```python
from build123d import *

# Parameters (mm, degrees)
SKETCH1_W                                       = 25
SKETCH1_H                                       = 51.4
BOSS_EXTRUDE1_DEPTH                             = 28.4
SKETCH2_W                                       = 47.3
SKETCH2_H                                       = 27.1
CUT_EXTRUDE1_DEPTH                              = 147
BOSS_EXTRUDE2_DEPTH                             = 11.9
BOSS_EXTRUDE2_DEPTH_BACK                        = 2
SKETCH4_W                                       = 25
SKETCH4_H                                       = 59.6
SKETCH5_W                                       = 55.6
SKETCH5_H                                       = 9.9
CUT_EXTRUDE5_DEPTH                              = 57.010088377
SKETCH6_W                                       = 51.6
SKETCH6_H                                       = 2
CUT_EXTRUDE6_DEPTH                              = 57.010088377
SKETCH7_W                                       = 25
SKETCH7_H                                       = 3
BOSS_EXTRUDE3_DEPTH                             = 15
SKETCH8_W                                       = 25
SKETCH8_H                                       = 3
BOSS_EXTRUDE4_DEPTH                             = 15
CSK_FOR_M3_FLAT_HEAD_MACHINE_SCREW4_D           = 3.4
CSK_FOR_M3_FLAT_HEAD_MACHINE_SCREW4_DEPTH       = 10.4
CSK_FOR_M3_FLAT_HEAD_MACHINE_SCREW4_CSINK_D     = 6.3
CSK_FOR_M3_FLAT_HEAD_MACHINE_SCREW4_CSINK_ANGLE = 90
CSK_FOR_M3_FLAT_HEAD_MACHINE_SCREW4_TIP         = 1.021463052


with BuildPart() as part:
    # Sketch1 → Boss-Extrude1 (new body)
    with BuildSketch(Plane(origin=(0, 0, 0), x_dir=(1, 0, 0), z_dir=(0, 1, 0))):
        Rectangle(SKETCH1_W, SKETCH1_H)
    extrude(amount=BOSS_EXTRUDE1_DEPTH)

    # Sketch2 → Cut-Extrude1 (cut)
    with BuildSketch(Plane(origin=(12.5, 0, 0), x_dir=(0, 0, -1), z_dir=(1, 0, 0))):
        with Locations((0, 12.55)):
            Rectangle(SKETCH2_W, SKETCH2_H)
    extrude(amount=-CUT_EXTRUDE1_DEPTH, mode=Mode.SUBTRACT)

    # Sketch4 → Boss-Extrude2 (add, two sides: drawn at the far end of the back side and taken through both)
    with BuildSketch(Plane(origin=(0, 28.4, 0), x_dir=(1, 0, 0), z_dir=(0, 1, 0)).offset(-BOSS_EXTRUDE2_DEPTH_BACK)):
        Rectangle(SKETCH4_W, SKETCH4_H)
    extrude(amount=BOSS_EXTRUDE2_DEPTH + BOSS_EXTRUDE2_DEPTH_BACK)

    # Sketch5 → Cut-Extrude5 (cut, through all)
    with BuildSketch(Plane.ZY.offset(12.5)):
        with Locations((0, 33.35)):
            Rectangle(SKETCH5_W, SKETCH5_H)
    extrude(amount=-CUT_EXTRUDE5_DEPTH, mode=Mode.SUBTRACT)

    # Sketch6 → Cut-Extrude6 (cut, through all)
    with BuildSketch(Plane.ZY.offset(12.5)):
        with Locations((0, 39.3)):
            Rectangle(SKETCH6_W, SKETCH6_H)
    extrude(amount=-CUT_EXTRUDE6_DEPTH, mode=Mode.SUBTRACT)

    # Sketch7 → Boss-Extrude3 (add)
    with BuildSketch(Plane(origin=(0, 0, -25.7), x_dir=(-1, 0, 0), z_dir=(0, 0, -1))):
        with Locations((0, 1.5)):
            Rectangle(SKETCH7_W, SKETCH7_H)
    extrude(amount=BOSS_EXTRUDE3_DEPTH)

    # Sketch8 → Boss-Extrude4 (add)
    with BuildSketch(Plane.XY.offset(25.7)):
        with Locations((0, 1.5)):
            Rectangle(SKETCH8_W, SKETCH8_H)
    extrude(amount=BOSS_EXTRUDE4_DEPTH)

    # CSK for M3 Flat Head Machine Screw4
    with Locations(Plane(origin=(0, 3, 0), x_dir=(1, 0, 0), z_dir=(0, 1, 0))):
        with Locations((0, 33.2), (0, -33.2)):
            CounterSinkHole(CSK_FOR_M3_FLAT_HEAD_MACHINE_SCREW4_D / 2, CSK_FOR_M3_FLAT_HEAD_MACHINE_SCREW4_CSINK_D / 2, depth=CSK_FOR_M3_FLAT_HEAD_MACHINE_SCREW4_DEPTH, counter_sink_angle=CSK_FOR_M3_FLAT_HEAD_MACHINE_SCREW4_CSINK_ANGLE)
            with Locations((0, 0, -(CSK_FOR_M3_FLAT_HEAD_MACHINE_SCREW4_DEPTH + CSK_FOR_M3_FLAT_HEAD_MACHINE_SCREW4_TIP / 2))):  # 118° drill point
                Cone(0, CSK_FOR_M3_FLAT_HEAD_MACHINE_SCREW4_D / 2, CSK_FOR_M3_FLAT_HEAD_MACHINE_SCREW4_TIP, mode=Mode.SUBTRACT)


solid = part.part
```
Check sheet for the modelled part. Datum: model origin and axes. Units: mm. A direction names the side the tool comes from. Give positions to 0.01 mm unless a question says otherwise; leave off trailing zeros. Order: outer loops, then holes, each group sorted by start corner. A loop starts at its lowest first (then second) coordinate and runs counter-clockwise, first axis right, second up. Notation, with made-up numbers: (-1.75, -39.75) -> (29.25, -39.75) arc R31 ccw to (29.25, -14.75) -> close; hole circle Ø6 at (71.25, 17.25). An arc over 180 degrees is marked (long way). Return JSON: item names as keys, results as strings.
1. Cross-section at A-A, the plane y = 23.5. Record the cut outline in (x, z), plus the area to 4 significant figures.
From the geometry:
{"outline": "(-12.5, -25.7) -> (12.5, -25.7) -> (12.5, -23.65) -> (-12.5, -23.65) -> close; (-12.5, 23.65) -> (12.5, 23.65) -> (12.5, 25.7) -> (-12.5, 25.7) -> close", "area": "102.5 mm^2"}
2. Go/stop test with flat-tipped pins: P1, Ø8, axis at x = -6.5, z = -20.5, coming from the +Y side; P2, Ø7, axis at x = 0, y = 33, coming from the -Z side; P3, Ø10, axis at x = 3, y = 17, coming from the +Z side. Record where each tip stops, or that it passes through.
From the geometry:
{"P1": "y = 28.4", "P2": "z = -29.8", "P3": "z = 25.7"}
3. Mould release check, pull along Z, two halves, no side actions. Record for faces 1 (the flat face through (0, 33, -27.8)), 2 (the flat face through (0, 2, 40.7)), 3 (the flat face through (0, 40.3, 28)): +Z half, -Z half, draft (parallel to the pull), parting line (faces both ways), or undercut.
From the geometry:
{"face 1": "undercut", "face 2": "+Z half", "face 3": "draft"}
4. Cross-section at C-C, the plane z = -33.2. Record the cut outline in (x, y).
From the geometry:
{"outline": "(-12.5, 0) -> (-1.7, 0) -> (-1.7, 1.55) -> (-3.15, 3) -> (-12.5, 3) -> close; (1.7, 0) -> (12.5, 0) -> (12.5, 3) -> (3.15, 3) -> (1.7, 1.55) -> close"}
5. Cross-section at D-D, the plane x = 0. Count the separate pieces of the cut face and the enclosed holes in it, plus the area to 3 significant figures.
From the geometry:
{"separate pieces": "3", "enclosed holes": "0", "area": "363 mm^2"}
6. Cross-section at B-B, the plane x = -5.75. Record the cut outline in (y, z).
From the geometry:
{"outline": "(0, -40.7) -> (3, -40.7) -> (3, -25.7) -> (26.4, -25.7) -> (26.4, -29.8) -> (40.3, -29.8) -> (40.3, -25.8) -> (38.3, -25.8) -> (38.3, -27.8) -> (28.4, -27.8) -> (28.4, 27.8) -> (38.3, 27.8) -> (38.3, 25.8) -> (40.3, 25.8) -> (40.3, 29.8) -> (26.4, 29.8) -> (26.4, 25.7) -> (3, 25.7) -> (3, 40.7) -> (0, 40.7) -> (0, 23.65) -> (26.1, 23.65) -> (26.1, -23.65) -> (0, -23.65) -> close"}
7. Set-up check for faces 4 (the flat face through (0, 33, -29.8)), 5 (the flat face through (0, 15, -25.7)), 6 (the flat face through (-3, 3, 35)), 7 (the flat face through (0, 38.3, -27)), 8 (the flat face through (0, 33, 29.8)): record each of +Z, -Z, +X, -X, +Y, -Y from which the full face is reachable in a straight line by a thin tool's end or side.
From the geometry:
{"face 4": "-Z, +X, -X, +Y", "face 5": "-Z, +X, -X", "face 6": "+Z, +X, -X", "face 7": "+X, -X", "face 8": "+Z, +X, -X, +Y"}
8. Material ranges on probe 1 along Z at (x, y) = (0, 1.05); probe 2 along X at (y, z) = (0.8, 33.2); probe 3 along Z at (x, y) = (-9.75, 17), recorded low to high. Write a range as [from, to].
From the geometry:
{"probe 1": "[-40.7, -34.9], [-31.5, -23.65], [23.65, 31.5], [34.9, 40.7]", "probe 2": "[-12.5, -1.7], [1.7, 12.5]", "probe 3": "[-25.7, -23.65], [23.65, 25.7]"}
